from build123d import *

# Parameters (mm, degrees)
BOSS_EXTRUDE1_DEPTH        = 10
BOSS_EXTRUDE1_DEPTH_BACK   = 2
SKETCH1_W                  = 0.5
SKETCH1_H                  = 0.5
BOSS_EXTRUDE1_2_DEPTH      = 10
BOSS_EXTRUDE1_2_DEPTH_BACK = 2
SKETCH2_R                  = 2
BOSS_EXTRUDE2_DEPTH        = 1
CUT_EXTRUDE1_DEPTH         = 3


with BuildPart() as part:
    # Sketch1 → Boss-Extrude1 (new, two sides: drawn at the far end of the back side and taken through both)
    with BuildSketch(Plane.XY.offset(-BOSS_EXTRUDE1_DEPTH_BACK)):
        with Locations((-0.25, -0.25)):
            Rectangle(SKETCH1_W, SKETCH1_H)
    extrude(amount=BOSS_EXTRUDE1_DEPTH + BOSS_EXTRUDE1_DEPTH_BACK)



with BuildPart() as body_2:
    # Sketch1 → Boss-Extrude1 2 (new, two sides: drawn at the far end of the back side and taken through both)
    with BuildSketch(Plane.XY.offset(-BOSS_EXTRUDE1_2_DEPTH_BACK)):
        with Locations((2.25, -0.25)):
            Rectangle(SKETCH1_W, SKETCH1_H)
    extrude(amount=BOSS_EXTRUDE1_2_DEPTH + BOSS_EXTRUDE1_2_DEPTH_BACK)


with BuildPart() as part_1:
    add(part.part)

    add(body_2.part)  # Boss-Extrude2 merges body 2
    # Sketch2 → Boss-Extrude2 (add)
    with BuildSketch(Plane.XY.offset(10)):
        with Locations((1, -0.25)):
            Circle(SKETCH2_R)
    extrude(amount=BOSS_EXTRUDE2_DEPTH)

    # Sketch5 → Cut-Extrude1 (cut)
    with BuildSketch(Plane(origin=(0, 0, 10), x_dir=(-1, 0, 0), z_dir=(0, 0, -1))):
        with BuildLine():
            Line((-2.322875656, -1.75), (0.322875656, -1.75))
            ThreePointArc((0.322875656, -1.75), (-1, -2.25), (-2.322875656, -1.75))
        make_face()
    extrude(amount=-CUT_EXTRUDE1_DEPTH, mode=Mode.SUBTRACT)

    # Sketch9 → Revolve6 (revolve)
    with BuildSketch(Plane(origin=(1, 0, 0), x_dir=(0, 0, -1), z_dir=(1, 0, 0)), mode=Mode.PRIVATE) as revolve6_sk:
        Polygon((-13.5, -0.251884355), (-13.998669849, -1.662558347), (-11, -1.751884355), (-11, -0.251884355), align=None)
    revolve(revolve6_sk.sketch.rotate(Axis((1, -0.251884355, 11), (0, 0, 1)), 180), axis=Axis((1, -0.251884355, 11), (0, 0, 1)))


solid = part_1.part
Here's how the part is built. I have some questions about the finished solid (model axes, mm). Give positions to 0.01 mm unless a question says otherwise; leave off trailing zeros. Write each loop counter-clockwise with the first axis right and the second up, starting at its lowest first coordinate (ties: lowest second). Pieces come first, ordered by that corner, then holes. Notation, with made-up numbers: (36.25, 14) -> (87.25, 14) arc R25 cw to (87.25, 43) -> close; hole circle Ø9 at (61, -6). An arc over 180 degrees is marked (long way). Use one line per item in the form item = value. Start each with the question number.
1. Will these pins go through, and if not, where does the flat tip stop? pin 1 Ø1.5 at (y, z) = (1.5, 5.5) entering from +X; pin 2 Ø0.6 at (x, z) = (-0.5, 4) entering from +Y; pin 3 Ø1 at (x, y) = (1.5, -0.5) entering from +Z; pin 4 Ø0.6 at (x, z) = (2.5, 2.5) entering from -Y.
2. Thinking about a two-plate mould opening in Y: for faces 1 (the face through (1.086, -0.271, 13.531)), 2 (the face through (1, 0, 10)), 3 (the face through (2.3, 0.4, 12.5)), which applies, +Y half, -Y half, draft (parallel to the pull), parting line (faces both ways), or undercut?
3. Imagine slicing it at B-B on x = -0.7. List the corners of the cut face in (y, z) for me, plus the area to 3 significant figures.
4. Imagine slicing it at A-A on z = -0.5. List the corners of the cut face in (x, y) for me.
5. If I drill on L1, parallel to X at y = -0.25, z = 3; L2, parallel to Y at x = -0.4, z = 9; L3, parallel to Z at x = 2.5, y = 1, over which ranges is the centre line in solid material (lowest first)?
6. Imagine slicing it at C-C on z = 11.5. List the corners of the cut face in (x, y) for me, plus the area to 3 significant figures.
Entries:
q1.pin_1 = through
q1.pin_2 = 0
q1.pin_3 = 13.87
q1.pin_4 = -0.5
q2.face_1 = undercut
q2.face_2 = draft
q2.face_3 = parting line
q3.outline = (-1.3, 10) -> (0.8, 10) -> (0.8, 11) -> (-1.3, 11) -> close
q3.area = 2.11 mm²
q4.outline = (-0.5, -0.5) -> (0, -0.5) -> (0, 0) -> (-0.5, 0) -> close; (2, -0.5) -> (2.5, -0.5) -> (2.5, 0) -> (2, 0) -> close
q5.L1 = -0.5 to 0, 2 to 2.5
q5.L2 = -0.5 to 0
q5.L3 = 10 to 11
q6.outline = circle Ø2.97 at (1, -0.25)
q6.area = 6.93 mm²
